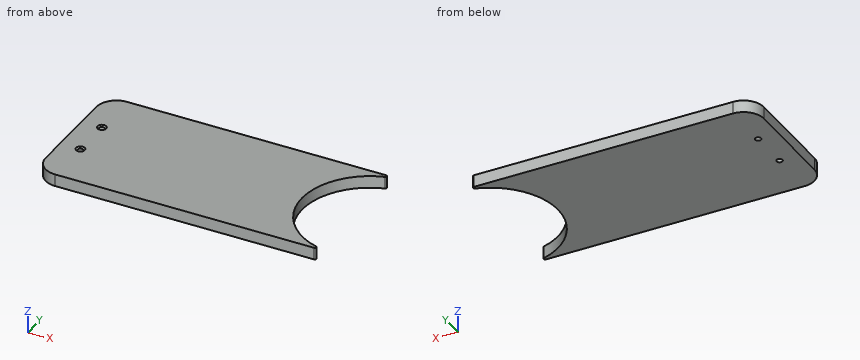
Autodesk Inventor part; units mm, degrees
ref_plane "YZ Plane" through (0, 0, 0) normal (1, 0, 0) x (0, 1, 0)
ref_plane "XZ Plane" through (0, 0, 0) normal (0, 1, 0) x (-1, 0, 0)
ref_plane "XY Plane" through (0, 0, 0) normal (0, 0, 1) x (1, 0, 0)
sketch "Эскиз1" plane through (0, 0, 0) normal (0, 0, 1) x (1, 0, 0)
  line L0 (51.75, 11.75) -> (0, 11.75)
  line L1 (0, -11.75) -> (51.75, -11.75)
  arc A0 (51.75, 11.75) -> (51.75, -11.75) centre (51.75, 0) ccw
  line L2 (0, -11.75) -> (0, 11.75)
  line L3 (0, 0) -> (40, 0) construction
  line L4 (0, 0) -> (0, 11.75) construction
  line L5 (0, 11.75) -> (0, 11.25)
  point P0 (20, 0)
  dimension "d0" = 11.75
  dimension "d47" = 40
extrude "Выдавливание3" add sketch "Эскиз1" along normal blind 2.1
fillet "Сопряжение3" radius 0.25 2 edges at (51.75, 11.75, 1.05) (51.75, -11.75, 1.05)
fillet "Сопряжение4" radius 3.5 2 edges at (0, -11.75, 1.05) (0, 11.75, 1.05)
sketch "Эскиз6" plane through (0, 0, 2.1) normal (0, 0, 1) x (1, 0, 0)
  arc A0 (48.3936, 11.2604) -> (48.3936, -11.2604) centre (51.75, 0) ccw construction
  line L0 (40, 0) -> (0, 0) construction
  line L1 (0, -11.75) -> (0, 11.75) construction
  circle A1 centre (3.5, 3.5) radius 0.5
  line L2 (3.5, 3.5) -> (0, 3.5) construction
  line L3 (3.5, 3.5) -> (3.5, 0) construction
  circle A2 centre (3.5, -3.5) radius 0.5
  point P0 (48.3222, -11.75)
  dimension "d58" = 1
  dimension "d59" = 3.5
hole "Отверстие1" at (3.5, -3.5, 2.1) at (3.5, 3.5, 2.1) direction (0, 0, -1) diameter 1 end through all countersink diameter 1.5 countersink angle 90
properties part number "Поршень"
Source: CAD feature listing. Evaluate the final solid. Frame: model axes, mm. Round coordinates to 2 decimals unless told otherwise and drop trailing zeros. Loops run counter-clockwise (first coordinate to the right, second up) from the corner with the lowest first, then second, coordinate; pieces in that order, holes last.
Q1. Ray query, line 1 (Y direction, x = 3.5, z = 0.45); line 2 (Y direction, x = 43, z = 1.7); line 3 (X direction, y = 3.25, z = 1.5). Return the intervals inside material, ascending.
Q2. First-contact query: P1, Ø10, axis at x = 17, y = 1, coming from the -Z side. Flat tip, straight axial feed; report the tip coordinate or a pass-through.
Q3. Section D-D, the plane y = 10.25. Return loops of the section in (x, z), plus the area to 3 significant figures.
Q4. Section C-C, the plane y = 1.5. Return loops of the section in (x, z), plus the area to 3 significant figures.
Q5. Section A-A, the plane z = 1.2. Return loops of the section in (x, y).
Q6. Section B-B, the plane y = -3.5. Return loops of the section in (x, z), plus the area to 3 significant figures.
Solutions:
1. line 1: y = -11.75 to -4, -3 to 3, 4 to 11.75
1. line 2: y = -11.75 to -7.84, 7.84 to 11.75
1. line 3: x = 0 to 3.07, 3.93 to 40.46
2. P1: stops at z = 0
3. outline: (0.63, 0) - (46.01, 0) - (46.01, 2.1) - (0.63, 2.1) - close
3. area: 95.3 mm2
4. outline: (0, 0) - (40.1, 0) - (40.1, 2.1) - (0, 2.1) - close
4. area: 84.2 mm2
5. outline: (0, -8.25) arc R3.5 ccw to (3.5, -11.75) - (48.32, -11.75) arc R0.25 ccw to (48.39, -11.26) arc R11.75 cw to (48.39, 11.26) arc R0.25 ccw to (48.32, 11.75) - (3.5, 11.75) arc R3.5 ccw to (0, 8.25) - close; hole circle Ø1 at (3.5, -3.5); hole circle Ø1 at (3.5, 3.5)
6. outline: (0, 0) - (3, 0) - (3, 1.85) - (2.75, 2.1) - (0, 2.1) - close; (4, 0) - (40.53, 0) - (40.53, 2.1) - (4.25, 2.1) - (4, 1.85) - close
6. area: 83.0 mm2
